Design review of the part built by this model. Coordinates are the model's own, in mm. Face numbers are marked on the shaded views. A direction names the side the tool comes from. Coordinates: 2 decimals unless noted, no trailing zeros. Order: outer loops, then holes, each group sorted by start corner. A loop starts at its lowest first (then second) coordinate and runs counter-clockwise, first axis right, second up. Notation, with made-up numbers: (19, 55.5) -> (70, 55.5) arc R13 cw to (70, 79.5) -> close; hole circle Ø11 at (28.25, 83.25). An arc over 180 degrees is marked (long way). Use a Markdown table: item, result. Add a question column.
Q1. Add section D-D (y = -22). State the section outline as (x, z) points, then the cut area to 3 significant figures.
Q2. Add section A-A (x = 6.5). State the section outline as (y, z) points.
Q3. Insertion check: pin 1 (1.9 mm diameter, centred on y = 34, z = 2, fed in from +X); pin 2 (3 mm diameter, centred on x = 35.5, z = 4.5, fed in from +Y); pin 3 (3 mm diameter, centred on y = 38.5, z = 4.5, fed in from -X). Each pin has a flat end and moves straight along its axis. Give the tip position at first contact, or say it passes through.
Q4. The part is to be moulded in two halves that separate along X. For the marked faces 5, 6 and 7, say which applies: pulls with the +X half, pulls with the -X half, needs draft (parallel to the pull), parting line crosses it, or undercut.
Q5. Add section C-C (z = 2.25). Count the separate pieces of the cut face and the enclosed holes in it, then the cut area to 3 significant figures.
Q6. Machinability: for the marked faces 1, 2, 3 and 4, which of the approach directions +Z, -Z, +X, -X, +Y, -Y give a long, thin tool a straight path to every point of the face, cutting with its end or side? Answer none if there is none.
Q7. Add section B-B (y = 34). State the section outline as (x, z) points, then the cut area to 3 significant figures.
Q8. Wall thickness on probe 1 along Y at (x, z) = (-1, 2.25); probe 2 along X at (y, z) = (31.5, 4.5); probe 3 along X at (y, z) = (-37, 4.5): over which ranges is each line inside the solid? List them lowest first.
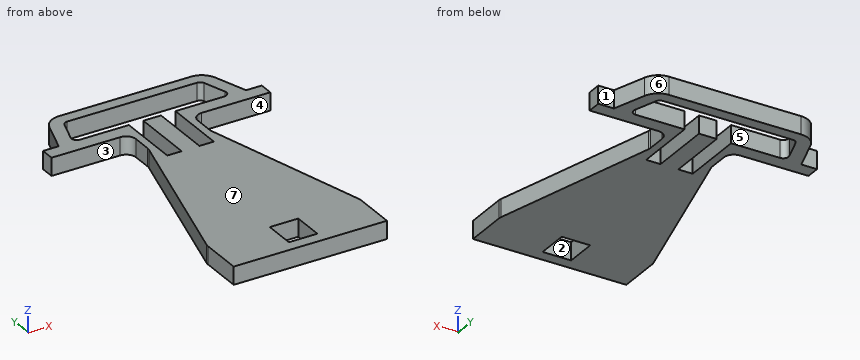
from build123d import *

# Parameters (mm, degrees)
F1_DEPTH = 6.35


with BuildPart() as f1:
    # F0 (on Top) → F1 (new body)
    with BuildSketch(Plane.XY):
        with BuildLine():
            ThreePointArc((-33.4219, 43.115239), (-32.867102, 41.775839), (-31.527702, 41.221041))
            Line((-31.527702, 41.221041), (-25.33034, 41.221041))
            Line((-25.33034, 41.221041), (-14.553085, 41.221041))
            ThreePointArc((-14.553085, 41.221041), (-12.062966, 40.1896), (-11.031525, 37.699481))
            Line((-11.031525, 37.699481), (-11.031525, 30.911574))
            ThreePointArc((-11.031525, 30.911574), (-11.061958, 30.449601), (-11.152732, 29.995613))
            Line((-11.152732, 29.995613), (-27.223983, -29.666242))
            ThreePointArc((-27.223983, -29.666242), (-27.314757, -30.12023), (-27.34519, -30.582203))
            Line((-27.34519, -30.582203), (-27.34519, -45.643087))
            Line((-27.34519, -45.643087), (0, -45.643087))
            Line((0, -45.643087), (27.34519, -45.643087))
            Line((27.34519, -45.643087), (27.34519, -30.582203))
            ThreePointArc((27.34519, -30.582203), (27.314757, -30.12023), (27.223983, -29.666242))
            Line((27.223983, -29.666242), (11.152732, 29.995613))
            ThreePointArc((11.152732, 29.995613), (11.061958, 30.449601), (11.031525, 30.911574))
            Line((11.031525, 30.911574), (11.031525, 37.699481))
            ThreePointArc((11.031525, 37.699481), (12.062966, 40.1896), (14.553085, 41.221041))
            Line((14.553085, 41.221041), (25.33034, 41.221041))
            Line((25.33034, 41.221041), (31.527702, 41.221041))
            ThreePointArc((31.527702, 41.221041), (32.867102, 41.775839), (33.4219, 43.115239))
            Line((33.4219, 43.115239), (33.4219, 46.182986))
            Line((33.4219, 46.182986), (29.585455, 57.798627))
            ThreePointArc((29.585455, 57.798627), (27.275806, 60.953424), (23.555821, 62.157143))
            Line((23.555821, 62.157143), (0, 62.157143))
            Line((0, 62.157143), (-23.555821, 62.157143))
            ThreePointArc((-23.555821, 62.157143), (-27.275806, 60.953424), (-29.585455, 57.798627))
            Line((-29.585455, 57.798627), (-33.4219, 46.182986))
            Line((-33.4219, 46.182986), (-33.4219, 43.115239))
        make_face()
        Polygon((-5.088463, -30.357072), (0, -30.357072), (5.088463, -30.357072), (5.088463, -41.450173), (0, -41.450173), (-5.088463, -41.450173), align=None, mode=Mode.SUBTRACT)
        with BuildLine():
            Line((-8.303855, 46.301041), (-25.737514, 46.301041))
            ThreePointArc((-25.737514, 46.301041), (-27.272644, 47.085572), (-27.536148, 48.789297))
            Line((-27.536148, 48.789297), (-24.933654, 56.66889))
            ThreePointArc((-24.933654, 56.66889), (-24.244688, 57.609963), (-23.135021, 57.969031))
            Line((-23.135021, 57.969031), (0, 57.969031))
            Line((0, 57.969031), (23.135021, 57.969031))
            ThreePointArc((23.135021, 57.969031), (24.244688, 57.609963), (24.933654, 56.66889))
            Line((24.933654, 56.66889), (27.531461, 48.803486))
            ThreePointArc((27.531461, 48.803486), (27.266455, 47.090046), (25.722571, 46.301041))
            Line((25.722571, 46.301041), (8.303855, 46.301041))
            Line((8.303855, 46.301041), (8.303855, 23.983043))
            Line((8.303855, 23.983043), (3.15923, 23.983043))
            Line((3.15923, 23.983043), (3.15923, 46.301041))
            Line((3.15923, 46.301041), (0, 46.301041))
            Line((0, 46.301041), (-3.15923, 46.301041))
            Line((-3.15923, 46.301041), (-3.15923, 23.983043))
            Line((-3.15923, 23.983043), (-8.303855, 23.983043))
            Line((-8.303855, 23.983043), (-8.303855, 46.301041))
        make_face(mode=Mode.SUBTRACT)
        with BuildLine():
            Line((-39.013032, 41.221041), (-31.527702, 41.221041))
            ThreePointArc((-31.527702, 41.221041), (-32.867102, 41.775839), (-33.4219, 43.115239))
            Line((-33.4219, 43.115239), (-33.4219, 46.182986))
            Line((-33.4219, 46.182986), (-39.013032, 46.182986))
            Line((-39.013032, 46.182986), (-39.013032, 41.221041))
        make_face()
        with BuildLine():
            Line((39.013032, 46.182986), (33.4219, 46.182986))
            Line((33.4219, 46.182986), (33.4219, 43.115239))
            ThreePointArc((33.4219, 43.115239), (32.867102, 41.775839), (31.527702, 41.221041))
            Line((31.527702, 41.221041), (39.013032, 41.221041))
            Line((39.013032, 41.221041), (39.013032, 46.182986))
        make_face()
    extrude(amount=F1_DEPTH)


solid = f1.part
Established:
| question | item | result |
|---|---|---|
| 1 | outline | (-25.16, 0) -> (25.16, 0) -> (25.16, 6.35) -> (-25.16, 6.35) -> close |
| 1 | area | 320 mm^2 |
| 2 | outline | (-45.64, 0) -> (23.98, 0) -> (23.98, 6.35) -> (-45.64, 6.35) -> close; (57.97, 0) -> (62.16, 0) -> (62.16, 6.35) -> (57.97, 6.35) -> close |
| 3 | pin 1 | x = 11.03 |
| 3 | pin 2 | y = 46.18 |
| 3 | pin 3 | x = -11.89 |
| 4 | face 5 | undercut |
| 4 | face 6 | pulls with the +X half |
| 4 | face 7 | needs draft |
| 5 | separate pieces | 1 |
| 5 | enclosed holes | 2 |
| 5 | area | 3,820 mm^2 |
| 6 | face 1 | +Z, -Z, +X, +Y |
| 6 | face 2 | +Z, -Z |
| 6 | face 3 | +Z, -Z, -X |
| 6 | face 4 | +Z, -Z, +X |
| 7 | outline | (-11.03, 0) -> (-8.3, 0) -> (-8.3, 6.35) -> (-11.03, 6.35) -> close; (-3.16, 0) -> (3.16, 0) -> (3.16, 6.35) -> (-3.16, 6.35) -> close; (8.3, 0) -> (11.03, 0) -> (11.03, 6.35) -> (8.3, 6.35) -> close |
| 7 | area | 74.8 mm^2 |
| 8 | probe 1 | -45.64 to -41.45, -30.36 to 46.3, 57.97 to 62.16 |
| 8 | probe 2 | -11.03 to -8.3, -3.16 to 3.16, 8.3 to 11.03 |
| 8 | probe 3 | -27.35 to -5.09, 5.09 to 27.35 |
